Check sheet for the modelled part. Datum: model origin and axes. Units: mm. A direction names the side the tool comes from. Give positions to 0.01 mm unless a question says otherwise; leave off trailing zeros. Write each loop counter-clockwise with the first axis right and the second up, starting at its lowest first coordinate (ties: lowest second). Pieces come first, ordered by that corner, then holes. Notation, with made-up numbers: (83.25, -17) -> (89.25, -17) arc R22 ccw to (89.25, 4) -> close; hole circle Ø1 at (23.25, 64.5). An arc over 180 degrees is marked (long way). Write each question's results on one line, items separated by ' | '. Start each with the question number.
```python
from build123d import *

# Parameters (mm, degrees)
CROQUIS2_W              = 995
CROQUIS2_H              = 654
SALIENTE_EXTRUIR1_DEPTH = 20
CROQUIS4_W              = 895
CROQUIS4_H              = 595
SALIENTE_EXTRUIR2_DEPTH = 75
CROQUIS6_W              = 851
CROQUIS6_H              = 560.386984293
CORTAR_EXTRUIR1_DEPTH   = 67
CROQUIS7_W              = 55
CROQUIS7_H              = 50
SALIENTE_EXTRUIR3_DEPTH = 880
CROQUIS9_W              = 55
CROQUIS9_H              = 50
SALIENTE_EXTRUIR5_DEPTH = 880
CROQUIS10_W             = 55
CROQUIS10_H             = 50
SALIENTE_EXTRUIR6_DEPTH = 880
CROQUIS11_W             = 55
CROQUIS11_H             = 50
SALIENTE_EXTRUIR7_DEPTH = 880
CROQUIS14_W             = 895
CROQUIS14_H             = 20
EXTRUIR_L_MINA4_DEPTH   = 596
CROQUIS22_W             = 895
CROQUIS22_H             = 595
SALIENTE_EXTRUIR8_DEPTH = 65
CROQUIS25_W             = 851
CROQUIS25_H             = 495
CORTAR_EXTRUIR2_DEPTH   = 65
CROQUIS26_W             = 785
CROQUIS26_H             = 552
CORTAR_EXTRUIR3_DEPTH   = 65


with BuildPart() as part:
    # Croquis2 → Saliente-Extruir1 (new body)
    with BuildSketch(Plane(origin=(0, 0, 0), x_dir=(1, 0, 0), z_dir=(0, 1, 0))):
        with Locations((0.447794779, -19.364986499)):
            Rectangle(CROQUIS2_W, CROQUIS2_H)
    extrude(amount=SALIENTE_EXTRUIR1_DEPTH)

    # Croquis4 → Saliente-Extruir2 (add)
    with BuildSketch(Plane(origin=(0, 0, 0), x_dir=(1, 0, 0), z_dir=(0, 1, 0))):
        with Locations((-4.552205221, -19.364986499)):
            Rectangle(CROQUIS4_W, CROQUIS4_H)
    extrude(amount=SALIENTE_EXTRUIR2_DEPTH)

    # Croquis6 → Cortar-Extruir1 (cut)
    with BuildSketch(Plane(origin=(0, 75, 0), x_dir=(1, 0, 0), z_dir=(0, 1, 0))):
        with Locations((-4.552205221, -24.058478646)):
            Rectangle(CROQUIS6_W, CROQUIS6_H)
    extrude(amount=-CORTAR_EXTRUIR1_DEPTH, mode=Mode.SUBTRACT)

    # Croquis7 → Saliente-Extruir3 (add)
    with BuildSketch(Plane(origin=(0, 0, 0), x_dir=(1, 0, 0), z_dir=(0, 1, 0))):
        with Locations((-424.552205221, -291.864986499)):
            Rectangle(CROQUIS7_W, CROQUIS7_H)
    extrude(amount=SALIENTE_EXTRUIR3_DEPTH)

    # Croquis9 → Saliente-Extruir5 (add)
    with BuildSketch(Plane(origin=(0, 0, 0), x_dir=(1, 0, 0), z_dir=(0, 1, 0))):
        with Locations((-424.552205221, 253.135013501)):
            Rectangle(CROQUIS9_W, CROQUIS9_H)
    extrude(amount=SALIENTE_EXTRUIR5_DEPTH)

    # Croquis10 → Saliente-Extruir6 (add)
    with BuildSketch(Plane(origin=(0, 0, 0), x_dir=(1, 0, 0), z_dir=(0, 1, 0))):
        with Locations((415.447794779, 253.135013501)):
            Rectangle(CROQUIS10_W, CROQUIS10_H)
    extrude(amount=SALIENTE_EXTRUIR6_DEPTH)

    # Croquis11 → Saliente-Extruir7 (add)
    with BuildSketch(Plane(origin=(0, 0, 0), x_dir=(1, 0, 0), z_dir=(0, 1, 0))):
        with Locations((415.447794779, -291.864986499)):
            Rectangle(CROQUIS11_W, CROQUIS11_H)
    extrude(amount=SALIENTE_EXTRUIR7_DEPTH)

    # Croquis14 → Extruir-Lámina4 (add)
    with BuildSketch(Plane.XY.offset(316.864986499)):
        with Locations((-4.552205221, 595)):
            Rectangle(CROQUIS14_W, CROQUIS14_H)
    extrude(amount=-EXTRUIR_L_MINA4_DEPTH)

    # Croquis22 → Saliente-Extruir8 (add)
    with BuildSketch(Plane(origin=(0, 605, 0), x_dir=(1, 0, 0), z_dir=(0, 1, 0))):
        with Locations((-4.552205221, -19.364986499)):
            Rectangle(CROQUIS22_W, CROQUIS22_H)
    extrude(amount=SALIENTE_EXTRUIR8_DEPTH)

    # Croquis25 → Cortar-Extruir2 (cut)
    with BuildSketch(Plane(origin=(0, 670, 0), x_dir=(1, 0, 0), z_dir=(0, 1, 0))):
        with Locations((-4.552205221, -19.364986499)):
            Rectangle(CROQUIS25_W, CROQUIS25_H)
    extrude(amount=-CORTAR_EXTRUIR2_DEPTH, mode=Mode.SUBTRACT)

    # Croquis26 → Cortar-Extruir3 (cut)
    with BuildSketch(Plane(origin=(0, 670, 0), x_dir=(1, 0, 0), z_dir=(0, 1, 0))):
        with Locations((-4.552205221, -18.864986499)):
            Rectangle(CROQUIS26_W, CROQUIS26_H)
    extrude(amount=-CORTAR_EXTRUIR3_DEPTH, mode=Mode.SUBTRACT)


solid = part.part
```
Item 1: Section check A-A on y = 115.5. Record the boundary of the cut face in (x, z), then the cut area to 3 significant figures.
Item 2: Depth check by flat-ended pin: pin 1 Ø2 at (x, z) = (52.5, -68.5) entering from +Y; pin 2 Ø4 at (y, z) = (638, 152) entering from +X; pin 3 Ø25 at (y, z) = (752.5, -255) entering from -X; pin 4 Ø8 at (x, z) = (-217, 125) entering from -Y. Enter the tip coordinate at first touch or a pass-through.
Item 3: Set-up check for faces 1 (the flat face through (-397.052, 741, -253)), 2 (the flat face through (-452.052, 635, 23)), 3 (the flat face through (-430.052, 42, 23)), 4 (the flat face through (-73, 607, 316.865)): record each of +Z, -Z, +X, -X, +Y, -Y from which the full face is reachable in a straight line by a thin tool's end or side.
Item 4: Section check C-C on x = -208. Record the boundary of the cut face in (y, z).
Item 5: Thickness scan on probe 1 along Y at (x, z) = (48.5, 185); probe 2 along Z at (x, y) = (-305.5, 60); probe 3 along X at (y, z) = (620.5, -30). Record the ranges inside material, lowest first. Write a range as from..to.
Item 6: Mould release check, pull along Y, two halves, no side actions. Record for faces 5 (the flat face through (415, 292, 266.865)), 6 (the flat face through (-425, 741, 266.865)), 7 (the flat face through (-425, 880, -253)): pulls with the +Y half, pulls with the -Y half, needs draft (parallel to the pull), parting line crosses it, or undercut.
Item 7: Section check B-B on z = -171. Record the boundary of the cut face in (x, y).
Check sheet entries:
1) outline: (-452.05, -278.14) -> (-397.05, -278.14) -> (-397.05, -228.14) -> (-452.05, -228.14) -> close; (-452.05, 266.86) -> (-397.05, 266.86) -> (-397.05, 316.86) -> (-452.05, 316.86) -> close; (387.95, -278.14) -> (442.95, -278.14) -> (442.95, -228.14) -> (387.95, -228.14) -> close; (387.95, 266.86) -> (442.95, 266.86) -> (442.95, 316.86) -> (387.95, 316.86) -> close | area: 11,000 mm^2
2) pin 1: stops at y = 605 | pin 2: stops at x = 442.95 | pin 3: stops at x = -452.05 | pin 4: stops at y = 0
3) face 1: +Y | face 2: +Z, -Z, -X, +Y | face 3: none | face 4: +Z, +X, -X, +Y
4) outline: (0, -307.64) -> (20, -307.64) -> (20, -278.14) -> (75, -278.14) -> (75, -256.14) -> (8, -256.14) -> (8, 304.25) -> (75, 304.25) -> (75, 316.86) -> (20, 316.86) -> (20, 346.36) -> (0, 346.36) -> close; (585, -279.14) -> (605, -279.14) -> (605, -278.14) -> (670, -278.14) -> (670, -257.14) -> (605, -257.14) -> (605, 294.86) -> (670, 294.86) -> (670, 316.86) -> (585, 316.86) -> close
5) probe 1: y = 0..8, 585..605 | probe 2: z = -278.14..-256.14, 304.25..316.86 | probe 3: x = -452.05..-430.05, 420.95..442.95
6) face 5: undercut | face 6: needs draft | face 7: pulls with the +Y half
7) outline: (-497.05, 0) -> (497.95, 0) -> (497.95, 20) -> (442.95, 20) -> (442.95, 75) -> (420.95, 75) -> (420.95, 8) -> (-430.05, 8) -> (-430.05, 75) -> (-452.05, 75) -> (-452.05, 20) -> (-497.05, 20) -> close; (-452.05, 585) -> (442.95, 585) -> (442.95, 670) -> (420.95, 670) -> (420.95, 605) -> (-430.05, 605) -> (-430.05, 670) -> (-452.05, 670) -> close
